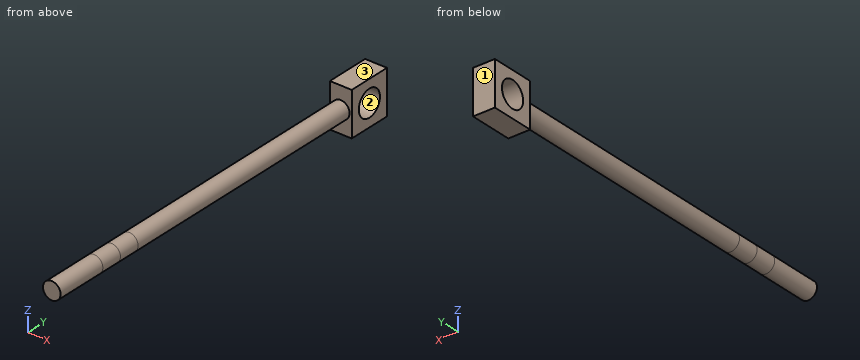
```python
from build123d import *

# Parameters (mm, degrees)
SKETCH_1_R       = 2
EXTRUDE_1_DEPTH  = 60
SKETCH_8_W       = 10
SKETCH_8_H       = 10
SKETCH_8_R       = 3
EXTRUDE_8_DEPTH  = 2.5
EXTRUDE_START    = 5
SKETCH_9_R       = 2
EXTRUDE_9_DEPTH  = 5
SKETCH_12_R      = 2
EXTRUDE_11_DEPTH = 5
EXTRUDE_START_2  = 7
SKETCH_10_R      = 2
EXTRUDE_10_DEPTH = 12


with BuildPart() as part:
    # Sketch 1 → Extrude 1 (new body)
    with BuildSketch(Plane(origin=(0, 0, 0), x_dir=(1, 0, 0), z_dir=(0, 1, 0))):
        with Locations(Location((0, 0, 0), (0, 0, 270))):
            Circle(SKETCH_1_R)
    extrude(amount=EXTRUDE_1_DEPTH)

    # Sketch 8 → Extrude 8 (add, symmetric)
    with BuildSketch(Plane(origin=(0, 0, 0), x_dir=(0, 0, -1), z_dir=(1, 0, 0))):
        with Locations((0, 65)):
            Rectangle(SKETCH_8_W, SKETCH_8_H)
        with Locations((0, 65)):
            Circle(SKETCH_8_R, mode=Mode.SUBTRACT)
    extrude(amount=EXTRUDE_8_DEPTH, both=True)

    # Sketch 9 → Extrude 9 (add)
    with BuildSketch(Plane.XZ.offset(EXTRUDE_START)):
        with Locations(Location((0, 0, 0), (0, 0, 270))):
            Circle(SKETCH_9_R)
    extrude(amount=-EXTRUDE_9_DEPTH)

    # Sketch 12 → Extrude 11 (add)
    with BuildSketch(Plane.XZ.offset(5).offset(EXTRUDE_START)):
        with Locations(Location((0, 0, 0), (0, 0, 270))):
            Circle(SKETCH_12_R)
    extrude(amount=-EXTRUDE_11_DEPTH)

    # Sketch 10 → Extrude 10 (add)
    with BuildSketch(Plane.XZ.offset(15).offset(EXTRUDE_START_2)):
        with Locations(Location((0, 0, 0), (0, 0, 270))):
            Circle(SKETCH_10_R)
    extrude(amount=-EXTRUDE_10_DEPTH)


solid = part.part
```
Geometry: final body of the model. Coordinates: model frame, mm. Face numbers are marked on the shaded views. Round coordinates to 2 decimals unless told otherwise and drop trailing zeros. Order: outer loops, then holes, each group sorted by start corner. A loop starts at its lowest first (then second) coordinate and runs counter-clockwise, first axis right, second up. Notation, with made-up numbers: (86, 24.25) -> (115, 24.25) arc R14 cw to (115, 51.25) -> close; hole circle Ø5 at (2, 3.25). An arc over 180 degrees is marked (long way). Use CSV: the item, a comma, the result in double quotes. Start each with the question number.
1) Section C-C (y = 65). Return the cut outline in (x, z).
2) Material intervals for line 1 along Y through (x, z) = (-0.6, 0); line 2 along Y through (x, z) = (-0.75, 4); line 3 along Y through (x, z) = (-0.4, 0.75), sorted ascending. Write a range as from..to.
3) First-contact query: pin 1 Ø5 at (y, z) = (-10.5, 3) entering from -X; pin 2 Ø4 at (y, z) = (37, 3) entering from +X; pin 3 Ø1.5 at (y, z) = (-1, -3) entering from -X; pin 4 Ø6 at (y, z) = (44.5, -1) entering from +X. Flat tips, straight axial feed; report the tip coordinate or a pass-through.
4) Section A-A (x = 0). Return the cut outline in (y, z).
5) Section D-D (y = -15). Return the cut outline in (x, z).
6) Draft query along Z for the marked faces 1, 2 and 3. Return one class per face: +Z half, -Z half, draft (parallel to the pull), parting line (faces both ways), or undercut.
7) Section B-B (z = 0). Return the cut outline in (x, y).
Returned:
1,outline,"(-2.5, -5) -> (2.5, -5) -> (2.5, -3) -> (-2.5, -3) -> close; (-2.5, 3) -> (2.5, 3) -> (2.5, 5) -> (-2.5, 5) -> close"
2,line 1,"y = -22..62, 68..70"
2,line 2,"y = 60..70"
2,line 3,"y = -22..62.1, 67.9..70"
3,pin 1,"stops at x = -1.94"
3,pin 2,"stops at x = 1.73"
3,pin 3,"passes through"
3,pin 4,"stops at x = 2"
4,outline,"(-22, -2) -> (60, -2) -> (60, -5) -> (70, -5) -> (70, 5) -> (60, 5) -> (60, 2) -> (-22, 2) -> close; hole circle Ø6 at (65, 0)"
5,outline,"circle Ø4 at (0, 0)"
6,face 1,"draft"
6,face 2,"undercut"
6,face 3,"+Z half"
7,outline,"(-2.5, 60) -> (-2, 60) -> (-2, -22) -> (2, -22) -> (2, 60) -> (2.5, 60) -> (2.5, 62) -> (-2.5, 62) -> close; (-2.5, 68) -> (2.5, 68) -> (2.5, 70) -> (-2.5, 70) -> close"
